CAD build for the part. Positions are in the model's coordinates, mm. Face numbers are marked on the shaded views. A direction names the side the tool comes from. Round coordinates to 2 decimals unless told otherwise and drop trailing zeros. Order: outer loops, then holes, each group sorted by start corner. A loop starts at its lowest first (then second) coordinate and runs counter-clockwise, first axis right, second up.
```python
from build123d import *

# Parameters (mm, degrees)
F1_DEPTH = 38.1


with BuildPart() as f1:
    # F0 (on Front) → F1 (new body)
    with BuildSketch(Plane.XZ):
        with BuildLine():
            add(Edge.make_bspline(
                [(-124.698026, -38.298128), (-124.698026, -6.657428), (-109.722411, 97.596107), (-55.124661, 142.541462)],
                knots=[0, 0, 0, 0, 185.214936, 185.214936, 185.214936, 185.214936], degree=3))
            ThreePointArc((-124.698026, -38.298128), (-87.037867, -125.729423), (2.301974, -158.606644))
            ThreePointArc((2.301974, -158.606644), (91.641816, -125.729423), (129.301974, -38.298128))
            add(Edge.make_bspline(
                [(129.301974, -38.298128), (129.301974, 2.429356), (104.489639, 163.465356), (2.301974, 163.465356)],
                knots=[0, 0, 0, 0, 238.406173, 238.406173, 238.406173, 238.406173], degree=3))
            add(Edge.make_bspline(
                [(-46.119579, 149.159544), (-32.330696, 158.131419), (-16.295798, 163.465356), (2.301974, 163.465356)],
                knots=[195.017142, 195.017142, 195.017142, 195.017142, 238.406173, 238.406173, 238.406173, 238.406173], degree=3))
            Line((-46.119579, 149.159544), (-35.702314, 93.036128))
            Line((-35.702314, 93.036128), (-1.729349, 115.201356))
            Line((-1.729349, 115.201356), (-8.66785, -13.442805))
            Line((-8.66785, -13.442805), (-24.936882, 73.096852))
            Line((-24.936882, 73.096852), (-60.107851, 50.150001))
            Line((-60.107851, 50.150001), (-55.124661, 142.541462))
        make_face()
    extrude(amount=F1_DEPTH)


solid = f1.part
```
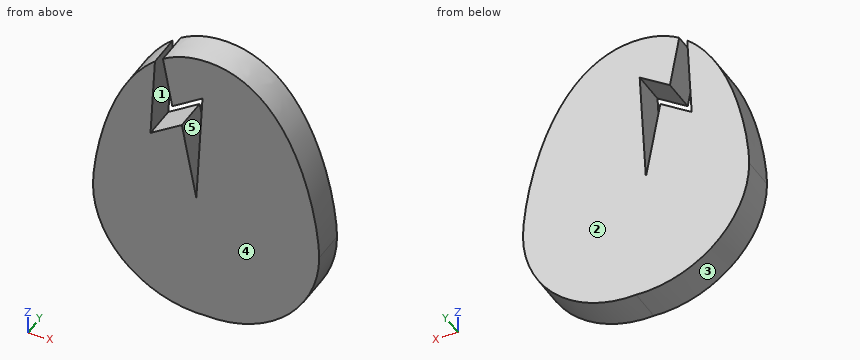
1. Tool access for the marked faces 1 and 2: list every direction of +Z, -Z, +X, -X, +Y, -Y with a clear straight run to the whole face (end or side of a thin tool).
2. Drill centre lines: line 1 (X direction, y = -12, z = 95); line 2 (X direction, y = -14.5, z = 62.5); line 3 (X direction, y = -35, z = 120). Where is each one in solid material? Low to high.
3. Cut at D-D, the plane z = -88.5. Write the cut outline in (x, y).
4. Pin check, flat tips, straight feed: P1, Ø12, axis at y = -14.5, z = -65, coming from the +X side; P2, Ø2, axis at x = -35, y = -7.5, coming from the +Z side; P3, Ø10, axis at y = -28.5, z = 1, coming from the +X side. Stop position of each tip, or through.
5. Cut at A-A, the plane z = 56. Give the number of separate pieces and of enclosed holes in the cut face, and give its area (3 significant figures).
6. Cut at B-B, the plane z = -134.5. Write the cut outline in (x, y).
7. Mould opens along Z. For the marked faces 3, 4 and 5 say: released by +Z, released by -Z, zero draft, split by the parting line, or undercut.
Outcome:
1. face 1: +Y, -Y
1. face 2: +Z, -Z, +X, -X, +Y
2. line 1: x = -91.56 to -57.69, -36.07 to -32.69, -2.82 to 96.17
2. line 2: x = -105.41 to -59.44, -41.18 to -22.94, -4.57 to 110.02
2. line 3: x = -76.19 to -56.34, -40.71 to 80.8
3. outline: (-113.7, -38.1) - (118.3, -38.1) - (118.3, 0) - (-113.7, 0) - close
4. P1: stops at x = 127.49
4. P2: stops at z = 155.8
4. P3: stops at x = 126.26
5. separate pieces: 3
5. enclosed holes: 0
5. area: 7,410 mm2
6. outline: (-76.67, -38.1) - (81.27, -38.1) - (81.27, 0) - (-76.67, 0) - close
7. face 3: released by -Z
7. face 4: zero draft
7. face 5: undercut
